The drawing under review shows one solid part. Ordinate dimensions are in mm from its lowest x, y, z. A direction names the side the tool comes from. Give positions to 0.01 mm unless a question says otherwise; leave off trailing zeros. Write each loop counter-clockwise with the first axis right and the second up, starting at its lowest first coordinate (ties: lowest second). Pieces come first, ordered by that corner, then holes. Notation, with made-up numbers: M 12,14 L 53,14 A24 cw 53,26 Z; hole C -14,-23 d1. An arc over 180 degrees is marked long. Answer as a JSON object with one key per item and string values. Group by question number.
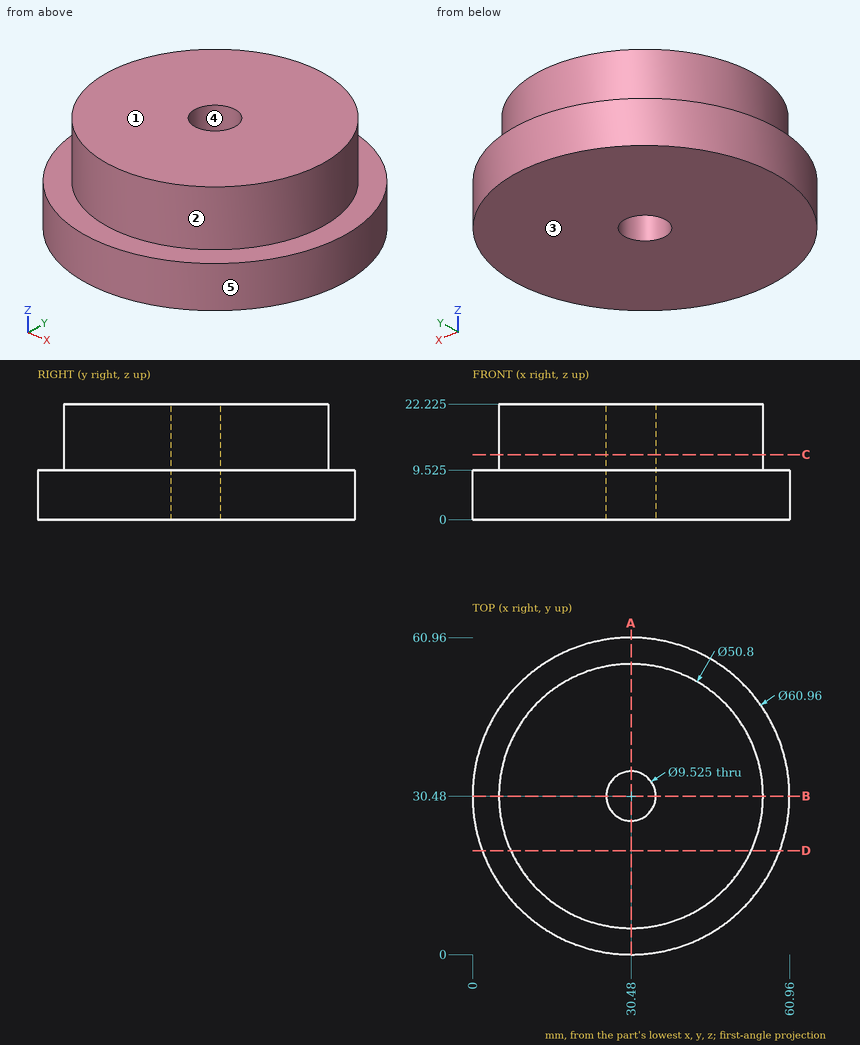
Item 1: Consider section D-D (y = 20). Give the boundary of the cut face in (x, z) (3 decimals), plus the area to 3 significant figures.
Item 2: Machinability: for the marked faces 1 and 2, which of the approach directions +Z, -Z, +X, -X, +Y, -Y give a long, thin tool a straight path to every point of the face, cutting with its end or side? Answer none if there is none.
Item 3: Consider section C-C (z = 12.5). Give the boundary of the cut face in (x, y) (1 decimal), plus the area to 3 significant figures.
Item 4: Insertion check: P1, Ø3, axis at y = 14, z = 5, coming from the +X side; P2, Ø4, axis at y = 36.5, z = 13, coming from the +X side; P3, Ø12, axis at y = 13, z = 19, coming from the +X side. Each pin has a flat end and moves straight along its axis. Give the tip position at first contact, or say it passes through.
Item 5: To check wall thickness, follow probe 1 along Y at (x, z) = (30.48, 8); probe 2 along Z at (x, y) = (57.5, 32) (3 decimals); probe 3 along Y at (x, z) = (30.48, 12.75). State the ranges of each line that lie inside material, in increasing order.
Item 6: Consider section A-A (x = 30.48). Give the boundary of the cut face in (y, z) (1 decimal).
Item 7: Draft analysis for pull direction X (two halves, no side actions). For the marked faces 3, 4 and 5, state which applies: released by +X, released by -X, zero draft, split by the parting line, or undercut.
Result set:
{
 "1": {"outline": "M 1.858,0 L 59.102,0 L 59.102,9.525 L 53.617,9.525 L 53.617,22.225 L 7.343,22.225 L 7.343,9.525 L 1.858,9.525 Z", "area": "1,130 mm^2"},
 "2": {"face 1": "+Z, +X, -X, +Y, -Y", "face 2": "+Z"},
 "3": {"outline": "C 30.5,30.5 d50.8; hole C 30.5,30.5 d9.5", "area": "1,960 mm^2"},
 "4": {"P1": "stops at x = 57.02", "P2": "stops at x = 55.56", "P3": "stops at x = 53.14"},
 "5": {"probe 1": "y = 0 to 25.72, 35.24 to 60.96", "probe 2": "z = 0 to 9.525", "probe 3": "y = 5.08 to 25.72, 35.24 to 55.88"},
 "6": {"outline": "M 0,0 L 25.7,0 L 25.7,22.2 L 5.1,22.2 L 5.1,9.5 L 0,9.5 Z; M 35.2,0 L 61,0 L 61,9.5 L 55.9,9.5 L 55.9,22.2 L 35.2,22.2 Z"},
 "7": {"face 3": "zero draft", "face 4": "undercut", "face 5": "split by the parting line"}
}
